CAD build for the part. Positions are in the model's coordinates, mm. Round coordinates to 2 decimals unless told otherwise and drop trailing zeros. Order: outer loops, then holes, each group sorted by start corner. A loop starts at its lowest first (then second) coordinate and runs counter-clockwise, first axis right, second up. Notation, with made-up numbers: M -26,56 L 11,56 A8 cw 11,70 Z; hole C 52.25,66 d1. An arc over 180 degrees is marked long. Answer as a JSON object with one key per item and string values.
```python
from build123d import *

# Parameters (mm, degrees)
SKETCH1_R           = 2.7
BOSS_EXTRUDE1_DEPTH = 5
FILLET1_R           = 10


with BuildPart() as part:
    # Sketch1 → Boss-Extrude1 (new body)
    with BuildSketch(Plane.XY):
        with BuildLine():
            Line((0, 0), (20, 0))
            Line((20, 0), (20, 5.3))
            Line((20, 5.3), (35.5, 5.3))
            Line((35.5, 5.3), (35.5, 0))
            Line((35.5, 0), (122.529437252, 0))
            Line((122.529437252, 0), (122.529437252, 5.3))
            Line((122.529437252, 5.3), (138.029437252, 5.3))
            Line((138.029437252, 5.3), (138.029437252, 0))
            Line((138.029437252, 0), (153.029437252, 0))
            Line((153.029437252, 0), (161.514718626, -8.485281374))
            ThreePointArc((161.514718626, -8.485281374), (170, -12), (178.485281374, -8.485281374))
            Line((178.485281374, -8.485281374), (186.970562748, 0))
            Line((186.970562748, 0), (201.970562748, 0))
            Line((201.970562748, 0), (201.970562748, 5.3))
            Line((201.970562748, 5.3), (217.470562748, 5.3))
            Line((217.470562748, 5.3), (217.470562748, 0))
            Line((217.470562748, 0), (304.5, 0))
            Line((304.5, 0), (304.5, 5.3))
            Line((304.5, 5.3), (320, 5.3))
            Line((320, 5.3), (320, 0))
            Line((320, 0), (345, 0))
            Line((345, 0), (345, 24))
            Line((345, 24), (0, 24))
            Line((0, 24), (0, 0))
        make_face()
        with Locations((170, 0)):
            Circle(SKETCH1_R, mode=Mode.SUBTRACT)
        with Locations((12, 12)):
            Circle(SKETCH1_R, mode=Mode.SUBTRACT)
        with Locations((333, 12)):
            Circle(SKETCH1_R, mode=Mode.SUBTRACT)
        with Locations((27.75, 14.65)):
            Circle(SKETCH1_R, mode=Mode.SUBTRACT)
        with Locations((130.279437252, 14.65)):
            Circle(SKETCH1_R, mode=Mode.SUBTRACT)
        with Locations((209.720562748, 14.65)):
            Circle(SKETCH1_R, mode=Mode.SUBTRACT)
        with Locations((312.25, 14.65)):
            Circle(SKETCH1_R, mode=Mode.SUBTRACT)
    extrude(amount=BOSS_EXTRUDE1_DEPTH)

    # Fillet1
    fillet1_edges = [part.edges().sort_by_distance(p)[0] for p in [
        (0, 24, 2.5),
        (345, 24, 2.5),
        (186.970562748, 0, 2.5),
        (153.029437252, 0, 2.5),
    ]]
    fillet(fillet1_edges, radius=FILLET1_R)


solid = part.part
```
Item 1: Wall check: line 1 along X through (y, z) = (5, 1.45); line 2 along Y through (x, z) = (12, 1.15); line 3 along Y through (x, z) = (312.25, 2.3). Give the ranges that are in metal, low to high. Write a range as [from, to].
Worked answers:
{"line 1": "x = [0, 20], [35.5, 122.53], [138.03, 201.97], [217.47, 304.5], [320, 345]", "line 2": "y = [0, 9.3], [14.7, 24]", "line 3": "y = [5.3, 11.95], [17.35, 24]"}
Item 2: Saw through at B-B on x = 236.5. List the corners of the cut face in (y, z), and give its area (3 significant figures).
Worked answers:
{"outline": "M 0,0 L 24,0 L 24,5 L 0,5 Z", "area": "120 mm2"}
Item 3: Saw through at A-A on z = 2.35. State how many separate pieces and enclosed holes the cut face has, and give its area (3 significant figures).
Worked answers:
{"separate pieces": "1", "enclosed holes": "7", "area": "8,010 mm2"}
Item 4: Drop flat-ended pins along their axis: pin 1 Ø2 at (x, z) = (288, 2.5) entering from -Y; pin 2 Ø1.5 at (x, z) = (206.5, 2) entering from -Y. Give the stop position or say it passes through.
Worked answers:
{"pin 1": "stops at y = 0", "pin 2": "stops at y = 5.3"}
Item 5: Two-plate mould, pull along X, no slides. Class faces 1 (the cylindrical face through (2.85, 20.99, 2.54)), 2 (the flat face through (181.22, -5.75, 2.46)), 3 (the cylindrical face through (314.744, 13.616, 2.465)): released by +X, released by -X, zero draft, split by the parting line, or undercut.
Worked answers:
{"face 1": "released by -X", "face 2": "released by +X", "face 3": "undercut"}
